from build123d import *

# Parameters (mm, degrees)
PAD_DEPTH     = 3.25
SKETCH001_R   = 4
SKETCH001_R_2 = 1.6
POCKET_DEPTH  = 3.5


with BuildPart() as part:
    # Sketch → Pad (new body)
    with BuildSketch(Plane.XY):
        with BuildLine():
            ThreePointArc((59.160798, -10), (0, 60), (-59.160798, -10))
            Line((-59.160798, -10), (-34.510465, -155.833333))
            ThreePointArc((-34.510465, -155.833333), (0, -185), (34.510465, -155.833333))
            Line((59.160798, -10), (34.510465, -155.833333))
        make_face()
    extrude(amount=PAD_DEPTH)

    # Sketch001 (on Face6 of Pad) → Pocket (cut)
    with BuildSketch(Plane.XY.offset(3.25)):
        with Locations((0, -150)):
            Circle(SKETCH001_R)
        with Locations((-7, -150)):
            Circle(SKETCH001_R_2)
        with Locations((7, -150)):
            Circle(SKETCH001_R_2)
        with Locations((0, -130)):
            Circle(SKETCH001_R)
        with Locations((7, -130)):
            Circle(SKETCH001_R_2)
        with Locations((-7, -130)):
            Circle(SKETCH001_R_2)
        with Locations((0, -140)):
            Circle(SKETCH001_R)
        with Locations((7, -140)):
            Circle(SKETCH001_R_2)
        with Locations((-7, -140)):
            Circle(SKETCH001_R_2)
        with Locations((0, -159.875452)):
            Circle(SKETCH001_R)
        with Locations((7, -159.875452)):
            Circle(SKETCH001_R_2)
        with Locations((-7, -159.875452)):
            Circle(SKETCH001_R_2)
        with Locations((0, -120)):
            Circle(SKETCH001_R)
        with Locations((7, -120)):
            Circle(SKETCH001_R_2)
        with Locations((-7, -120)):
            Circle(SKETCH001_R_2)
        with Locations((0, -110)):
            Circle(SKETCH001_R)
        with Locations((7, -110)):
            Circle(SKETCH001_R_2)
        with Locations((-7, -110)):
            Circle(SKETCH001_R_2)
    extrude(amount=-POCKET_DEPTH, mode=Mode.SUBTRACT)


solid = part.part
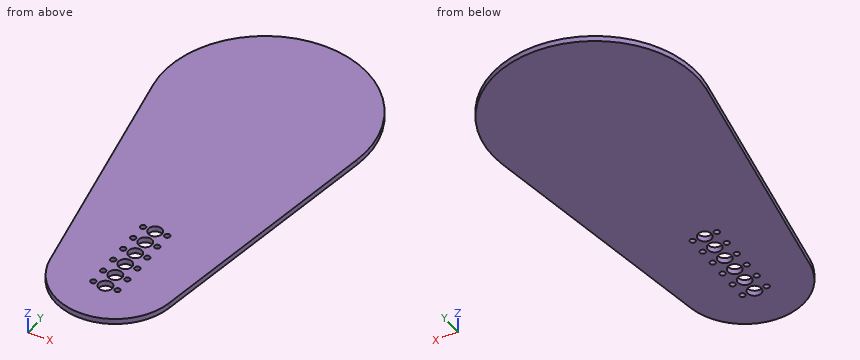
Model file for the job. Use its own axes, mm. Give positions to 0.01 mm unless a question says otherwise; leave off trailing zeros. Loops run counter-clockwise (first coordinate to the right, second up) from the corner with the lowest first, then second, coordinate; pieces in that order, holes last.
Item 1: Slice it at C-C (x = 40). Write the cut outline in (y, z).
Check values:
outline: (-123.36, 0) - (44.72, 0) - (44.72, 3.25) - (-123.36, 3.25) - close
Item 2: Slice it at B-B (y = -28). Write the cut outline in (x, z).
Check values:
outline: (-56.12, 0) - (56.12, 0) - (56.12, 3.25) - (-56.12, 3.25) - close
Item 3: Drop a flat-ended pin along its axis: P1, Ø1.9, axis at x = -7, y = -150, coming from the +Z side. Give the stop position or say it passes through.
Check values:
P1: passes through
Item 4: Slice it at A-A (z = 2.05). Give the number of separate pieces and of enclosed holes in the cut face, plus the area to 3 significant figures.
Check values:
separate pieces: 1
enclosed holes: 18
area: 21,600 mm2
Item 5: Drill centre lines: line 1 along X through (y, z) = (-105, 1); line 2 along X through (y, z) = (-45, 2.65); line 3 along Y through (x, z) = (31.5, 2.75). Where is each one in solid material? Low to high.
Check values:
line 1: x = -43.1 to 43.1
line 2: x = -53.24 to 53.24
line 3: y = -165.26 to 51.07
